```python
from build123d import *

# Parameters (mm, degrees)
F1_DEPTH = 12.7


with BuildPart() as f1:
    # F0 (on Front) → F1 (new body)
    with BuildSketch(Plane.XZ):
        Polygon((-120.65, 152.4), (-120.65, 139.7), (-139.7, 139.7), (-139.7, 120.65), (-152.4, 120.65), (-152.4, 107.95), (-139.7, 107.95), (-139.7, 95.25), (-152.4, 95.25), (-152.4, 82.55), (-139.7, 82.55), (-139.7, 69.85), (-152.4, 69.85), (-152.4, 57.15), (-139.7, 57.15), (-139.7, 44.45), (-152.4, 44.45), (-152.4, 31.75), (-139.7, 31.75), (-139.7, 19.05), (-152.4, 19.05), (-152.4, 6.35), (-139.7, 6.35), (-139.7, -6.35), (-152.4, -6.35), (-152.4, -19.05), (-139.7, -19.05), (-139.7, -31.75), (-152.4, -31.75), (-152.4, -44.45), (-139.7, -44.45), (-139.7, -57.15), (-152.4, -57.15), (-152.4, -69.85), (-139.7, -69.85), (-139.7, -82.55), (-152.4, -82.55), (-152.4, -95.25), (-139.7, -95.25), (-139.7, -107.95), (-152.4, -107.95), (-152.4, -120.65), (-139.7, -120.65), (-139.7, -139.7), (-120.65, -139.7), (-120.65, -152.4), (-107.95, -152.4), (-107.95, -139.7), (-95.25, -139.7), (-95.25, -152.4), (-82.55, -152.4), (-82.55, -139.7), (-69.85, -139.7), (-69.85, -152.4), (-57.15, -152.4), (-57.15, -139.7), (-44.45, -139.7), (-44.45, -152.4), (-31.75, -152.4), (-31.75, -139.7), (-19.05, -139.7), (-19.05, -152.4), (-6.35, -152.4), (-6.35, -139.7), (6.35, -139.7), (6.35, -152.4), (19.05, -152.4), (19.05, -139.7), (31.75, -139.7), (31.75, -152.4), (44.45, -152.4), (44.45, -139.7), (57.15, -139.7), (57.15, -152.4), (69.85, -152.4), (69.85, -139.7), (82.55, -139.7), (82.55, -152.4), (95.25, -152.4), (95.25, -139.7), (107.95, -139.7), (107.95, -152.4), (120.65, -152.4), (120.65, -139.7), (139.7, -139.7), (139.7, -120.65), (152.4, -120.65), (152.4, -107.95), (139.7, -107.95), (139.7, -95.25), (152.4, -95.25), (152.4, -82.55), (139.7, -82.55), (139.7, -69.85), (152.4, -69.85), (152.4, -57.15), (139.7, -57.15), (139.7, -44.45), (152.4, -44.45), (152.4, -31.75), (139.7, -31.75), (139.7, -19.05), (152.4, -19.05), (152.4, -6.35), (139.7, -6.35), (139.7, 6.35), (152.4, 6.35), (152.4, 19.05), (139.7, 19.05), (139.7, 31.75), (152.4, 31.75), (152.4, 44.45), (139.7, 44.45), (139.7, 57.15), (152.4, 57.15), (152.4, 69.85), (139.7, 69.85), (139.7, 82.55), (152.4, 82.55), (152.4, 95.25), (139.7, 95.25), (139.7, 107.95), (152.4, 107.95), (152.4, 120.65), (139.7, 120.65), (139.7, 139.7), (120.65, 139.7), (120.65, 152.4), (107.95, 152.4), (107.95, 139.7), (95.25, 139.7), (95.25, 152.4), (82.55, 152.4), (82.55, 139.7), (69.85, 139.7), (69.85, 152.4), (57.15, 152.4), (57.15, 139.7), (44.45, 139.7), (44.45, 152.4), (31.75, 152.4), (31.75, 139.7), (19.05, 139.7), (19.05, 152.4), (6.35, 152.4), (6.35, 139.7), (-6.35, 139.7), (-6.35, 152.4), (-19.05, 152.4), (-19.05, 139.7), (-31.75, 139.7), (-31.75, 152.4), (-44.45, 152.4), (-44.45, 139.7), (-57.15, 139.7), (-57.15, 152.4), (-69.85, 152.4), (-69.85, 139.7), (-82.55, 139.7), (-82.55, 152.4), (-95.25, 152.4), (-95.25, 139.7), (-107.95, 139.7), (-107.95, 152.4), align=None)
    extrude(amount=F1_DEPTH)


solid = f1.part
```
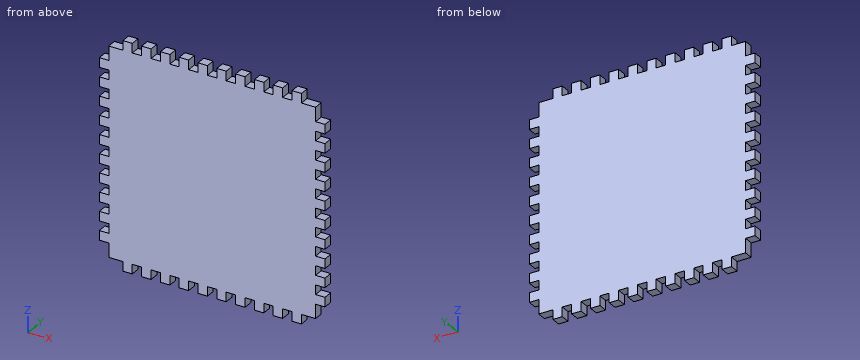
Check sheet for the modelled part. Datum: model origin and axes. Units: mm. Round coordinates to 2 decimals unless told otherwise and drop trailing zeros. Loops run counter-clockwise (first coordinate to the right, second up) from the corner with the lowest first, then second, coordinate; pieces in that order, holes last. Notation, with made-up numbers: (-7, 84) - (24, 84) arc R26 cw to (24, 116) - close; hole circle Ø2 at (-10.75, -4). An arc over 180 degrees is marked (long way). Answer as a JSON object with one key per item and string values. Group by question number.
Q1. Sectioned sample at A-A, the plane x = 104.5. Enter the section's corners in (y, z), plus the area to 3 significant figures.
Q2. Sectioned sample at B-B, the plane z = -125.5. Enter the section's corners in (x, y), plus the area to 3 significant figures.
Q3. Scan line: line 1 along Z through (x, y) = (56, -3.75). Record every from-to range of solid material in increasing order. Write a range as [from, to].
Q4. Gauge pin test, flat ends, axial feed: P1, Ø6.5, axis at x = 100.5, y = -6.5, coming from the -Z side; P2, Ø4, axis at x = -26.5, y = -5.5, coming from the +Z side; P3, Ø6.5, axis at y = -8.5, z = 144.5, coming from the -X side. Record the tip position at first contact, or that the pin passes through.
Solution:
{
 "1": {"outline": "(-12.7, -139.7) - (0, -139.7) - (0, 139.7) - (-12.7, 139.7) - close", "area": "3,550 mm²"},
 "2": {"outline": "(-139.7, -12.7) - (139.7, -12.7) - (139.7, 0) - (-139.7, 0) - close", "area": "3,550 mm²"},
 "3": {"line 1": "z = [-139.7, 139.7]"},
 "4": {"P1": "stops at z = -139.7", "P2": "stops at z = 139.7", "P3": "stops at x = -120.65"}
}
